from build123d import *

# Parameters (mm, degrees)
BOSS_EXTRUDE1_DEPTH = 20
SKETCH2_R           = 26
CUT_EXTRUDE1_DEPTH  = 40
FILLET1_R           = 5
CHAMFER1_SIZE       = 1
CHAMFER2_SIZE       = 5


with BuildPart() as part:
    # Sketch1 → Boss-Extrude1 (new, symmetric)
    with BuildSketch(Plane.XY):
        with BuildLine():
            Line((-276.915792692, 75), (73.084207308, 75))
            Line((73.084207308, 75), (73.084207308, 40))
            Line((73.084207308, 40), (-56.915792692, 40))
            Line((-56.915792692, 40), (-56.915792692, -40))
            Line((-56.915792692, -40), (73.084207308, -40))
            Line((73.084207308, -40), (73.084207308, -75))
            Line((73.084207308, -75), (-276.915792692, -75))
            ThreePointArc((-276.915792692, -75), (-346.915792692, 0), (-276.915792692, 75))
        make_face()
    extrude(amount=BOSS_EXTRUDE1_DEPTH, both=True)

    # Sketch2 → Cut-Extrude1 (cut)
    with BuildSketch(Plane.XY.offset(20)):
        with Locations((-276.915792692, 0)):
            Circle(SKETCH2_R)
    extrude(amount=-CUT_EXTRUDE1_DEPTH, mode=Mode.SUBTRACT)

    # Fillet1
    # the kernel refuses this fillet: 5 mm, written as the material it takes off along each edge
    with BuildSketch(Plane(origin=(78.084207308, -75, -20), x_dir=(0, 1, 0), z_dir=(-1, 0, 0)), Plane(origin=(-281.915792692, 75, 20), x_dir=(0, 0, -1), z_dir=(1, 0, 0))) as fillet1_piece_1:
        with BuildLine():
            CenterArc((FILLET1_R, -FILLET1_R), FILLET1_R, 90, 90)
            Line((0, -FILLET1_R), (-FILLET1_R * 0.02, -FILLET1_R))
            Line((-FILLET1_R * 0.02, -FILLET1_R), (-FILLET1_R * 0.02, FILLET1_R * 0.02))
            Line((-FILLET1_R * 0.02, FILLET1_R * 0.02), (FILLET1_R, FILLET1_R * 0.02))
            Line((FILLET1_R, FILLET1_R * 0.02), (FILLET1_R, 0))
        make_face()
    extrude(amount=360, mode=Mode.SUBTRACT)
    with BuildSketch(Plane(origin=(-271.737221263, 0, -20), x_dir=(-0.00233212005306246, -0.9999972806043315, 0), z_dir=(0.9999972806043315, -0.00233212005306246, 0))) as fillet1_piece_2:
        with BuildLine():
            CenterArc((75.178571429 - FILLET1_R, -FILLET1_R), FILLET1_R, 0, 90)
            Line((75.178571429 - FILLET1_R, 0), (75.178571429 - FILLET1_R, FILLET1_R * 0.02))
            Line((75.178571429 - FILLET1_R, FILLET1_R * 0.02), (75.178571429 + FILLET1_R * 0.02, FILLET1_R * 0.02))
            Line((75.178571429 + FILLET1_R * 0.02, FILLET1_R * 0.02), (75.178571429 + FILLET1_R * 0.02, -FILLET1_R))
            Line((75.178571429 + FILLET1_R * 0.02, -FILLET1_R), (75.178571429, -FILLET1_R))
        make_face()
    revolve(axis=Axis((-271.737221263, 0, -20), (0, 0, -1)), revolution_arc=179.732758485, mode=Mode.SUBTRACT)
    with BuildSketch(Plane(origin=(73.084207308, 75, 25), x_dir=(-1, 0, 0), z_dir=(0, 0, -1)), Plane(origin=(73.084207308, -75, -25), x_dir=(-1, 0, 0), z_dir=(0, 0, 1))) as fillet1_piece_3:
        with BuildLine():
            CenterArc((FILLET1_R, -FILLET1_R), FILLET1_R, 90, 90)
            Line((0, -FILLET1_R), (-FILLET1_R * 0.02, -FILLET1_R))
            Line((-FILLET1_R * 0.02, -FILLET1_R), (-FILLET1_R * 0.02, FILLET1_R * 0.02))
            Line((-FILLET1_R * 0.02, FILLET1_R * 0.02), (FILLET1_R, FILLET1_R * 0.02))
            Line((FILLET1_R, FILLET1_R * 0.02), (FILLET1_R, 0))
        make_face()
    extrude(amount=50, mode=Mode.SUBTRACT)
    with BuildSketch(Plane(origin=(-271.737221263, 0, 20), x_dir=(-0.00233212005306246, -0.9999972806043315, 0), z_dir=(0.9999972806043315, -0.00233212005306246, 0))) as fillet1_piece_4:
        with BuildLine():
            CenterArc((75.178571429 - FILLET1_R, FILLET1_R), FILLET1_R, 270, 90)
            Line((75.178571429 - FILLET1_R, 0), (75.178571429 - FILLET1_R, -FILLET1_R * 0.02))
            Line((75.178571429 - FILLET1_R, -FILLET1_R * 0.02), (75.178571429 + FILLET1_R * 0.02, -FILLET1_R * 0.02))
            Line((75.178571429 + FILLET1_R * 0.02, -FILLET1_R * 0.02), (75.178571429 + FILLET1_R * 0.02, FILLET1_R))
            Line((75.178571429 + FILLET1_R * 0.02, FILLET1_R), (75.178571429, FILLET1_R))
        make_face()
    revolve(axis=Axis((-271.737221263, 0, 20), (0, 0, -1)), revolution_arc=179.732758485, mode=Mode.SUBTRACT)
    with BuildSketch(Plane(origin=(78.084207308, -75, 20), x_dir=(0, 1, 0), z_dir=(-1, 0, 0)), Plane(origin=(-281.915792692, 75, -20), x_dir=(0, 0, 1), z_dir=(1, 0, 0))) as fillet1_piece_5:
        with BuildLine():
            CenterArc((FILLET1_R, FILLET1_R), FILLET1_R, 180, 90)
            Line((0, FILLET1_R), (-FILLET1_R * 0.02, FILLET1_R))
            Line((-FILLET1_R * 0.02, FILLET1_R), (-FILLET1_R * 0.02, -FILLET1_R * 0.02))
            Line((-FILLET1_R * 0.02, -FILLET1_R * 0.02), (FILLET1_R, -FILLET1_R * 0.02))
            Line((FILLET1_R, -FILLET1_R * 0.02), (FILLET1_R, 0))
        make_face()
    extrude(amount=360, mode=Mode.SUBTRACT)

    # Chamfer1
    chamfer1_edges = [part.edges().sort_by_distance(p)[0] for p in [
        (-302.915792692, 0, -20),
        (-302.915792692, 0, 20),
    ]]
    chamfer(chamfer1_edges, length=CHAMFER1_SIZE)

    # Chamfer2
    chamfer2_edges = [part.edges().sort_by_distance(p)[0] for p in [
        (8.084207308, -40, 20),
        (-56.915792692, 0, 20),
        (8.084207308, 40, 20),
        (8.084207308, 40, -20),
        (-56.915792692, 0, -20),
        (8.084207308, -40, -20),
    ]]
    chamfer(chamfer2_edges, length=CHAMFER2_SIZE)


solid = part.part
Geometry: final body of the model. Coordinates: model frame, mm. A direction names the side the tool comes from. Round coordinates to 2 decimals unless told otherwise and drop trailing zeros. Order: outer loops, then holes, each group sorted by start corner. A loop starts at its lowest first (then second) coordinate and runs counter-clockwise, first axis right, second up. Notation, with made-up numbers: (70.25, 1.25) -> (122.25, 1.25) arc R30 ccw to (122.25, 32.25) -> close; hole circle Ø11 at (65.5, -32). An arc over 180 degrees is marked (long way). Put each result on its own line as item: value. Start each with the question number.
Q1. Pull-direction query (X, two-part tool) for faces 1 (the flat face through (-56.916, 1, 0)), 2 (the cylindrical face through (-252.116, 7.81, 0.266)), 3 (the flat face through (9, 40, 0)); classes: +X half, -X half, draft (parallel to the pull), parting line (faces both ways), or undercut.
Q2. Reachability of faces 4 (the flat face through (7, -40, 0)), 5 (the flat face through (-102, -75, 0)) from +Z, -Z, +X, -X, +Y, -Y: full face, straight path, thin tool, end or side. Return the list, or none.
Q3. Section C-C on y = 0. Return the cut outline in (x, z), and give its area (3 significant figures).
Q4. First-contact query: pin 1 (5 mm diameter, centred on x = -93.5, z = 15.5, fed in from -Y); pin 2 (24 mm diameter, centred on y = 1.5, z = -5.5, fed in from +X); pin 3 (1.5 mm diameter, centred on y = 14, z = 15, fed in from -X). Flat tips, straight axial feed; report the tip coordinate or a pass-through.
Q5. Line query: probe 1 along Y at (x, z) = (-11.5, 4); probe 2 along Y at (x, z) = (-7.5, -17); probe 3 along X at (y, z) = (-6, -11.5). Output: solid intervals per line, ascending.
Q6. Section A-A on x = 28. Return the cut outline in (y, z).
Q7. Section B-B on z = 3.5. Return the cut outline in (x, y), and give its area (3 significant figures).
Ans:
1. face 1: +X half
1. face 2: undercut
1. face 3: draft
2. face 4: +Z, -Z, +X
2. face 5: +Z, -Z, +X, -X, -Y
3. outline: (-346.92, -15) arc R5 ccw to (-341.92, -20) -> (-303.92, -20) -> (-302.92, -19) -> (-302.92, 19) -> (-303.92, 20) -> (-341.92, 20) arc R5 ccw to (-346.92, 15) -> close; (-250.92, -19) -> (-249.92, -20) -> (-61.92, -20) -> (-56.92, -15) -> (-56.92, 15) -> (-61.92, 20) -> (-249.92, 20) -> (-250.92, 19) -> close
3. area: 9,480 mm2
4. pin 1: stops at y = -75
4. pin 2: stops at x = -56.92
4. pin 3: stops at x = -345.74
5. probe 1: y = -75 to -40, 40 to 75
5. probe 2: y = -74.58 to -42, 42 to 74.58
5. probe 3: x = -346.68 to -302.21, -251.62 to -56.92
6. outline: (-75, -15) arc R5 ccw to (-70, -20) -> (-45, -20) -> (-40, -15) -> (-40, 15) -> (-45, 20) -> (-70, 20) arc R5 ccw to (-75, 15) -> close; (40, -15) -> (45, -20) -> (70, -20) arc R5 ccw to (75, -15) -> (75, 15) arc R5 ccw to (70, 20) -> (45, 20) -> (40, 15) -> close
7. outline: (-276.92, -75) -> (68.08, -75) arc R5 ccw to (73.08, -70) -> (73.08, -40) -> (-56.92, -40) -> (-56.92, 40) -> (73.08, 40) -> (73.08, 70) arc R5 ccw to (68.08, 75) -> (-276.92, 75) arc R75.18 ccw to start; hole circle Ø52 at (-276.92, 0)
7. area: 48,100 mm2
